from build123d import *

# Parameters (mm, degrees)
SKETCH1_W           = 52
SKETCH1_H           = 40
BOSS_EXTRUDE1_DEPTH = 6
FILLET1_R           = 1
SKETCH2_W           = 48
SKETCH2_H           = 36
CUT_EXTRUDE1_DEPTH  = 10
SKETCH3_W           = 16
SKETCH3_H           = 46
BOSS_EXTRUDE2_DEPTH = 3
FILLET2_R           = 2
SKETCH4_R           = 5
CUT_EXTRUDE2_DEPTH  = 1
SKETCH5_W           = 3
SKETCH5_H           = 6
BOSS_EXTRUDE3_DEPTH = 1


with BuildPart() as part:
    # Sketch1 → Boss-Extrude1 (new, symmetric)
    with BuildSketch(Plane.XY):
        Rectangle(SKETCH1_W, SKETCH1_H)
    extrude(amount=BOSS_EXTRUDE1_DEPTH, both=True)

    # Fillet1
    fillet1_edges = [part.edges().sort_by_distance(p)[0] for p in [
        (-26, 20, 0),
        (26, 20, 0),
        (26, -20, 0),
        (-26, -20, 0),
    ]]
    fillet(fillet1_edges, radius=FILLET1_R)

    # Sketch2 → Cut-Extrude1 (cut)
    with BuildSketch(Plane.XY.offset(6)):
        with Locations((0, 1)):
            Rectangle(SKETCH2_W, SKETCH2_H)
    extrude(amount=-CUT_EXTRUDE1_DEPTH, mode=Mode.SUBTRACT)

    # Sketch3 → Boss-Extrude2 (add)
    with BuildSketch(Plane(origin=(26.00000007, 0, 0), x_dir=(0, 0, -1), z_dir=(1, 0, 0))):
        Rectangle(SKETCH3_W, SKETCH3_H)
    extrude(amount=BOSS_EXTRUDE2_DEPTH)

    # Fillet2
    fillet2_edges = [part.edges().sort_by_distance(p)[0] for p in [
        (27.50000007, 23, 8),
        (27.50000007, -23, 8),
        (27.50000007, -23, -8),
        (27.50000007, 23, -8),
    ]]
    fillet(fillet2_edges, radius=FILLET2_R)

    # Sketch4 → Cut-Extrude2 (cut)
    with BuildSketch(Plane(origin=(29.00000007, 0, 0), x_dir=(0, 0, -1), z_dir=(1, 0, 0))):
        Circle(SKETCH4_R)
    extrude(amount=-CUT_EXTRUDE2_DEPTH, mode=Mode.SUBTRACT)

    # Sketch5 → Boss-Extrude3 (add)
    with BuildSketch(Plane.ZY.offset(26)):
        with Locations((0, 8)):
            Rectangle(SKETCH5_W, SKETCH5_H)
        with Locations((0, -8)):
            Rectangle(SKETCH5_W, SKETCH5_H)
    extrude(amount=BOSS_EXTRUDE3_DEPTH)


solid = part.part
The model under review builds one solid part; all positions refer to its coordinate system, in mm. A direction names the side the tool comes from. Round coordinates to 2 decimals unless told otherwise and drop trailing zeros. Write each loop counter-clockwise with the first axis right and the second up, starting at its lowest first coordinate (ties: lowest second). Pieces come first, ordered by that corner, then holes. Notation, with made-up numbers: (37.25, 41) -> (74.25, 41) arc R27 ccw to (74.25, 75) -> close; hole circle Ø9 at (33, 87). An arc over 180 degrees is marked (long way). Answer as a JSON object with one key per item and string values.
1. We need section B-B on z = -0.5. State the section outline as (x, y) points.
Results found:
{"outline": "(-27, -11) -> (-26, -11) -> (-26, -19) arc R1 ccw to (-25, -20) -> (25, -20) arc R1 ccw to (26, -19) -> (26, -23) -> (29, -23) -> (29, -4.97) -> (28, -4.97) -> (28, 4.97) -> (29, 4.97) -> (29, 23) -> (26, 23) -> (26, 19) arc R1 ccw to (25, 20) -> (-25, 20) arc R1 ccw to (-26, 19) -> (-26, 11) -> (-27, 11) -> (-27, 5) -> (-26, 5) -> (-26, -5) -> (-27, -5) -> close; hole (-24, -17) -> (24, -17) -> (24, 19) -> (-24, 19) -> close"}
2. We need section C-C on x = -10. State the section outline as (y, z) points.
Results found:
{"outline": "(-20, -6) -> (20, -6) -> (20, 6) -> (19, 6) -> (19, -4) -> (-17, -4) -> (-17, 6) -> (-20, 6) -> close"}
3. We need section D-D on y = -13. State the section outline as (x, z) points, and give its area (3 significant figures).
Results found:
{"outline": "(-26, -6) -> (26, -6) -> (26, -8) -> (29, -8) -> (29, 8) -> (26, 8) -> (26, 6) -> (24, 6) -> (24, -4) -> (-24, -4) -> (-24, 6) -> (-26, 6) -> close", "area": "192 mm^2"}
4. Clearance check with flat-ended pins moving along their axes: pin 1 (12 mm diameter, centred on x = -18.5, y = 4, fed in from -Z); pin 2 (5 mm diameter, centred on x = -8, y = -11.5, fed in from +Z); pin 3 (5 mm diameter, centred on x = 5, z = 3.5, fed in from +Y). State where each tip first meets the part, or that it passes through.
Results found:
{"pin 1": "stops at z = -6", "pin 2": "stops at z = -4", "pin 3": "stops at y = 20"}
5. To check wall thickness, follow line 1 along X through (y, z) = (13.5, -3.75); line 2 along X through (y, z) = (-2, -3.75); line 3 along Y through (x, z) = (28.5, 0). State the ranges of each line that lie inside material, in increasing order.
Results found:
{"line 1": "x = -26 to -24, 24 to 29", "line 2": "x = -26 to -24, 24 to 28", "line 3": "y = -23 to -5, 5 to 23"}
6. Machinability: for faces 1 (the face through (0, 19, 1)), 2 (the face through (0, -20, 0)), 3 (the face through (0, 0, -6)), which of the approach directions +Z, -Z, +X, -X, +Y, -Y give a long, thin tool a straight path to every point of the face, cutting with its end or side? Answer none if there is none.
Results found:
{"face 1": "+Z", "face 2": "+Z, -Z, -X, -Y", "face 3": "-Z, -X, +Y, -Y"}
7. We need section A-A on y = 0. State the section outline as (x, z) points, and give its area (3 significant figures).
Results found:
{"outline": "(-26, -6) -> (26, -6) -> (26, -8) -> (29, -8) -> (29, -5) -> (28, -5) -> (28, 5) -> (29, 5) -> (29, 8) -> (26, 8) -> (26, 6) -> (24, 6) -> (24, -4) -> (-24, -4) -> (-24, 6) -> (-26, 6) -> close", "area": "182 mm^2"}
8. The part is to be moulded in two halves that separate along Y. For faces 4 (the face through (28, 0, 0)), 5 (the face through (24, 1, 1)), 6 (the face through (0, -18, 6)), 7 (the face through (27, -23, 0)), say which applies: pulls with the +Y half, pulls with the -Y half, needs draft (parallel to the pull), parting line crosses it, or undercut.
Results found:
{"face 4": "undercut", "face 5": "undercut", "face 6": "needs draft", "face 7": "pulls with the -Y half"}
